Here's how the part is built. I have some questions about the finished solid (model axes, mm). Give positions to 0.01 mm unless a question says otherwise; leave off trailing zeros. Write each loop counter-clockwise with the first axis right and the second up, starting at its lowest first coordinate (ties: lowest second). Pieces come first, ordered by that corner, then holes. Notation, with made-up numbers: M 48.25,72.5 L 88.25,72.5 A25 cw 88.25,102.5 Z; hole C 61.25,51.5 d9. An arc over 180 degrees is marked long. Use one line per item in the form item = value. Start each with the question number.
from build123d import *

# Parameters (mm, degrees)
SKETCH1_R                       = 55
BOSS_EXTRUDE1_DEPTH             = 3
SKETCH2_W                       = 70
SKETCH2_H                       = 100
BOSS_EXTRUDE2_DEPTH             = 3
BOSS_EXTRUDE3_DEPTH             = 3
SKETCH4_R                       = 46
CUT_EXTRUDE2_DEPTH              = 1
CUT_EXTRUDE2_DEPTH_BACK         = 4
CUT_EXTRUDE5_START              = -4
CUT_EXTRUDE5_DEPTH              = 5
CUT_EXTRUDE3_START              = -4
SKETCH5_R                       = 2.25
CUT_EXTRUDE3_DEPTH              = 5
CIRPATTERN1_COUNT               = 12
CUT_EXTRUDE4_START              = -4
SKETCH6_R                       = 3.25
CUT_EXTRUDE4_DEPTH              = 5
LPATTERN1_COUNT                 = 3
LPATTERN1_PITCH                 = 20
CUT_EXTRUDE6_START              = -1
SKETCH8_R                       = 2.25
CUT_EXTRUDE6_DEPTH              = 5
CIRPATTERN2_COUNT               = 3
CIRPATTERN2_ANGLE               = 20
CIRPATTERN2_THE_OTHER_WAY_COUNT = 3
CIRPATTERN2_THE_OTHER_WAY_ANGLE = 20


with BuildPart() as part:
    # Sketch1 → Boss-Extrude1 (new body)
    with BuildSketch(Plane(origin=(0, 0, 0), x_dir=(1, 0, 0), z_dir=(0, 1, 0))):
        Circle(SKETCH1_R)
    extrude(amount=BOSS_EXTRUDE1_DEPTH)

    # Sketch2 → Boss-Extrude2 (add)
    with BuildSketch(Plane(origin=(0, 0, 0), x_dir=(1, 0, 0), z_dir=(0, 1, 0))):
        with Locations((0, 92.426406871)):
            Rectangle(SKETCH2_W, SKETCH2_H)
    extrude(amount=BOSS_EXTRUDE2_DEPTH)

    # Sketch9 → Boss-Extrude3 (add)
    with BuildSketch(Plane(origin=(0, 0, 0), x_dir=(1, 0, 0), z_dir=(0, 1, 0))):
        Polygon((-35, 114.721305974), (-52.984880526, 14.751353687), (-17.871452142, 14.751353687), align=None)
    boss_extrude3 = extrude(amount=BOSS_EXTRUDE3_DEPTH)

    # Mirror2: Boss-Extrude3 across plane
    add(boss_extrude3.mirror(Plane(origin=(0, 0, 0), x_dir=(0, 0, 1), z_dir=(1, 0, 0))))

    # Sketch4 → Cut-Extrude2 (cut, two sides)
    with BuildSketch(Plane(origin=(0, 3, 0), x_dir=(1, 0, 0), z_dir=(0, 1, 0))) as cut_extrude2_sk:
        Circle(SKETCH4_R)
    extrude(amount=CUT_EXTRUDE2_DEPTH, mode=Mode.SUBTRACT)
    extrude(cut_extrude2_sk.sketch, amount=-CUT_EXTRUDE2_DEPTH_BACK, mode=Mode.SUBTRACT)

    # Sketch7 → Cut-Extrude5 (cut)
    with BuildSketch(Plane(origin=(0, 3, 0), x_dir=(1, 0, 0), z_dir=(0, 1, 0)).offset(CUT_EXTRUDE5_START)):
        with BuildLine():
            Line((0, 0), (0, -55))
            ThreePointArc((0, -55), (-24.969477486, -49.00535883), (-44.495934691, -32.328188876))
            Line((-44.495934691, -32.328188876), (0, 0))
        make_face()
    cut_extrude5 = extrude(amount=CUT_EXTRUDE5_DEPTH, mode=Mode.SUBTRACT)

    # Mirror1: Cut-Extrude5 across plane
    add(cut_extrude5.mirror(Plane(origin=(0, 0, 0), x_dir=(0, 0, 1), z_dir=(1, 0, 0))), mode=Mode.SUBTRACT)

    # Sketch5 → Cut-Extrude3 (cut)
    with BuildSketch(Plane(origin=(0, 3, 0), x_dir=(1, 0, 0), z_dir=(0, 1, 0)).offset(CUT_EXTRUDE3_START)):
        with Locations((0, 51)):
            Circle(SKETCH5_R)
    cut_extrude3 = extrude(amount=CUT_EXTRUDE3_DEPTH, mode=Mode.SUBTRACT)

    # CirPattern1: Cut-Extrude3 ×12 about axis
    cirpattern1_axis = Axis((0, 0, 0), (0, 1, 0))
    for i in range(1, CIRPATTERN1_COUNT):
        add(cut_extrude3.rotate(cirpattern1_axis, i * 360 / CIRPATTERN1_COUNT), mode=Mode.SUBTRACT)

    # Sketch6 → Cut-Extrude4 (cut)
    with BuildSketch(Plane(origin=(0, 3, 0), x_dir=(1, 0, 0), z_dir=(0, 1, 0)).offset(CUT_EXTRUDE4_START)):
        with Locations((15, 122.426406871)):
            Circle(SKETCH6_R)
        with Locations((-15, 122.426406871)):
            Circle(SKETCH6_R)
    cut_extrude4 = extrude(amount=CUT_EXTRUDE4_DEPTH, mode=Mode.SUBTRACT)

    # LPattern1: Cut-Extrude4 ×3
    with Locations(*[(0, 0, i * LPATTERN1_PITCH) for i in range(1, LPATTERN1_COUNT)]):
        add(cut_extrude4, mode=Mode.SUBTRACT)

    # Sketch8 → Cut-Extrude6 (cut)
    with BuildSketch(Plane(origin=(0, 0, 0), x_dir=(1, 0, 0), z_dir=(0, 1, 0)).offset(CUT_EXTRUDE6_START)):
        with Locations((0, 66.5)):
            Circle(SKETCH8_R)
    cut_extrude6 = extrude(amount=CUT_EXTRUDE6_DEPTH, mode=Mode.SUBTRACT)

    # CirPattern2: Cut-Extrude6 ×3 about axis
    cirpattern2_axis = Axis((0, 0, 0), (0, 1, 0))
    for i in range(1, CIRPATTERN2_COUNT):
        add(cut_extrude6.rotate(cirpattern2_axis, i * CIRPATTERN2_ANGLE / (CIRPATTERN2_COUNT - 1)), mode=Mode.SUBTRACT)

    # CirPattern2 the other way: Cut-Extrude6 ×3 about axis
    cirpattern2_the_other_way_axis = Axis((0, 0, 0), (0, -1, 0))
    for i in range(1, CIRPATTERN2_THE_OTHER_WAY_COUNT):
        add(cut_extrude6.rotate(cirpattern2_the_other_way_axis, i * CIRPATTERN2_THE_OTHER_WAY_ANGLE / (CIRPATTERN2_THE_OTHER_WAY_COUNT - 1)), mode=Mode.SUBTRACT)


solid = part.part
1) Suppose I cut it at B-B, the plane z = 0. List the corners of the cut face in (x, y) for me, and give its area (3 significant figures).
2) Suppose I cut it at C-C, the plane y = 2.3. State how many separate pieces and enclosed holes the cut face has, and give its area (3 significant figures).
3) Will this pin go through, and if not, where does the flat tip stop? P1, Ø3.5, axis at x = -51, z = 0, coming from the +Y side.
4) Suppose I cut it at D-D, the plane z = -51. List the corners of the cut face in (x, y) for me.
5) Thinking about a two-plate mould opening in Z: for faces 1 (the face through (-40.906, 1.479, 29.72)), 2 (the face through (-43.867, 1.479, -65.436)), 3 (the face through (-11.647, 1.479, -63.242)), 4 (the face through (-0.488, 1.479, -64.304)), which applies, released by +Z, released by -Z, zero draft, split by the parting line, or undercut?
6) Suppose I cut it at A-A, the plane x = 0. List the corners of the cut face in (y, z) for me, and give its area (3 significant figures).
7) Please list where these lines run through material, in increasing order: line 1 (Z direction, x = 0, y = 1.7); line 2 (X direction, y = 0.85, z = -63.5); line 3 (X direction, y = 0.2, z = -26).
Checks:
q1.outline = M -55,0 L -53.25,0 L -53.25,3 L -55,3 Z; M -48.75,0 L -46,0 L -46,3 L -48.75,3 Z; M 46,0 L 48.75,0 L 48.75,3 L 46,3 Z; M 53.25,0 L 55,0 L 55,3 L 53.25,3 Z
q1.area = 27.0 mm^2
q2.separate_pieces = 1
q2.enclosed_holes = 20
q2.area = 9,160 mm^2
q3.P1 = through
q4.outline = M -46.46,0 L -2.25,0 L -2.25,3 L -46.46,3 Z; M 2.25,0 L 46.46,0 L 46.46,3 L 2.25,3 Z
q5.face_1 = released by +Z
q5.face_2 = released by -Z
q5.face_3 = undercut
q5.face_4 = undercut
q6.outline = M 0,-142.43 L 3,-142.43 L 3,-68.75 L 0,-68.75 Z; M 0,-64.25 L 3,-64.25 L 3,-53.25 L 0,-53.25 Z; M 0,-48.75 L 3,-48.75 L 3,-46 L 0,-46 Z
q6.area = 262 mm^2
q7.line_1 = -142.43 to -68.75, -64.25 to -53.25, -48.75 to -46
q7.line_2 = -44.21 to -24.75, -20.73 to -12.6, -10.5 to 10.5, 12.6 to 20.73, 24.75 to 44.21
q7.line_3 = -50.96 to -46.36, -41.97 to -37.95, 37.95 to 41.97, 46.36 to 50.96
